Design review of the part shown in the three views and the two pictorial views. Dimensions are in mm from the part's minimum x, y and z. A direction names the side the tool comes from. Round coordinates to 2 decimals unless told otherwise and drop trailing zeros. Write each loop counter-clockwise with the first axis right and the second up, starting at its lowest first coordinate (ties: lowest second). Pieces come first, ordered by that corner, then holes. Notation, with made-up numbers: (-25, 37.25) -> (-2, 37.25) arc R21 ccw to (-2, 63.25) -> close; hole circle Ø2 at (52, -36.75). An arc over 180 degrees is marked (long way). Return JSON: item names as keys, results as strings. Group by question number.
1. Take a section at A-A, the plane y = 7. Write out the cut boundary in (x, z).
2. Take a section at C-C, the plane x = 7. Write out the cut boundary in (y, z), then the cut area to 3 significant figures.
3. Take a section at D-D, the plane z = 4.75. Write out the cut boundary in (x, y).
4. Mouldability with a two-part tool opening along X and no side actions: class the marked faces 1, 2 and 3 as pulls with the +X half, pulls with the -X half, needs draft (parallel to the pull), parting line crosses it, or undercut.
5. Tool access review of the marked faces 4, 5 and 6: name each direction out of +Z, -Z, +X, -X, +Y, -Y from which nothing blocks a thin tool from reaching the whole face with its end or side.
6. For line 1 along Z through (x, y) = (7, 12.3); line 2 along Z through (x, y) = (12.75, 5.5); line 3 along Y through (x, z) = (7, 6), list the stretches that pass through material, from the lowest coordinate up. Write a range as from..to.
7. Take a section at B-B, the plane y = 12.25. Write out the cut boundary in (x, z), then the cut area to 3 significant figures.
8. Clearance check with flat-ended pins moving along their axes: P1, Ø2, axis at x = 3.5, z = 2, coming from the +Y side; P2, Ø8, axis at x = 12, z = 7.5, coming from the +Y side; P3, Ø1.5, axis at y = 11.5, z = 10, coming from the -X side. State where each tip first meets the part, or that it passes through.
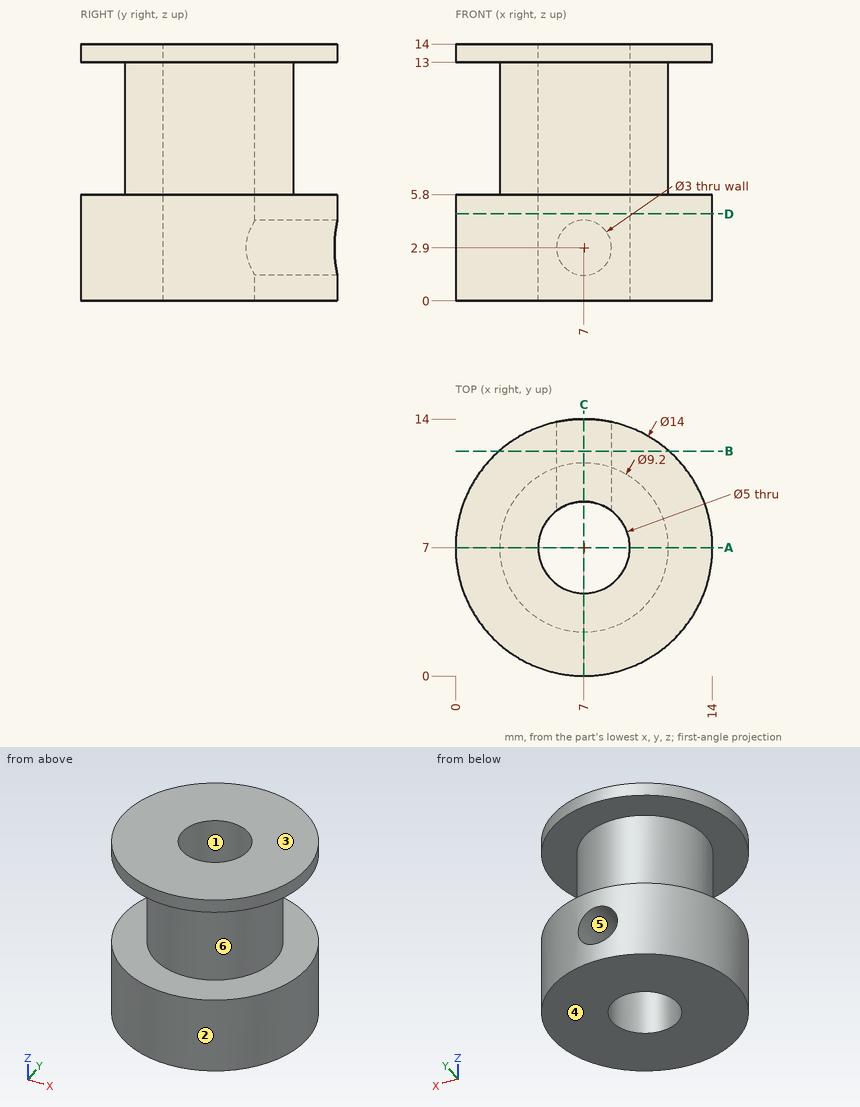
Output:
{
 "1": {"outline": "(0, 0) -> (4.5, 0) -> (4.5, 14) -> (0, 14) -> (0, 13) -> (2.4, 13) -> (2.4, 5.8) -> (0, 5.8) -> close; (9.5, 0) -> (14, 0) -> (14, 5.8) -> (11.6, 5.8) -> (11.6, 13) -> (14, 13) -> (14, 14) -> (9.5, 14) -> close"},
 "2": {"outline": "(0, 0) -> (4.5, 0) -> (4.5, 14) -> (0, 14) -> (0, 13) -> (2.4, 13) -> (2.4, 5.8) -> (0, 5.8) -> close; (9.5, 0) -> (14, 0) -> (14, 1.4) -> (9.5, 1.4) -> close; (9.5, 4.4) -> (14, 4.4) -> (14, 5.8) -> (11.6, 5.8) -> (11.6, 13) -> (14, 13) -> (14, 14) -> (9.5, 14) -> close", "area": "77.9 mm^2"},
 "3": {"outline": "circle Ø14 at (7, 7); hole circle Ø5 at (7, 7)"},
 "4": {"face 1": "undercut", "face 2": "parting line crosses it", "face 3": "needs draft"},
 "5": {"face 4": "-Z, +X, -X, +Y, -Y", "face 5": "+Y", "face 6": "none"},
 "6": {"line 1": "z = 0..1.4, 4.4..5.8, 13..14", "line 2": "z = 0..5.8, 13..14", "line 3": "y = 2.4..4.5, 9.5..11.6"},
 "7": {"outline": "(2.37, 0) -> (11.63, 0) -> (11.63, 5.8) -> (2.37, 5.8) -> close; (2.37, 13) -> (11.63, 13) -> (11.63, 14) -> (2.37, 14) -> close; hole circle Ø3 at (7, 2.9)", "area": "55.9 mm^2"},
 "8": {"P1": "stops at y = 13.54", "P2": "stops at y = 13.86", "P3": "stops at x = 4.34"}
}
